```python
from build123d import *

# Parameters (mm, degrees)
SKETCH1_W           = 18
SKETCH1_H           = 14
SKETCH1_R           = 0.5
BOSS_EXTRUDE1_DEPTH = 1
SKETCH2_R           = 4.15
BOSS_EXTRUDE2_DEPTH = 3.75
SKETCH3_W           = 4.05
SKETCH3_H           = 8.25
BOSS_EXTRUDE3_DEPTH = 4.4
SKETCH4_W           = 7.25
SKETCH4_H           = 2
SKETCH4_W_2         = 5.65
SKETCH4_H_2         = 0.9
CUT_EXTRUDE1_DEPTH  = 3
SKETCH5_R           = 3
CUT_EXTRUDE2_DEPTH  = 0.5
CHAMFER1_SIZE       = 0.5


with BuildPart() as part:
    # Sketch1 → Boss-Extrude1 (new body)
    with BuildSketch(Plane(origin=(0, 0, 0), x_dir=(1, 0, 0), z_dir=(0, 1, 0))):
        with Locations((9, 7)):
            Rectangle(SKETCH1_W, SKETCH1_H)
        with Locations(Location((16.5, 12.5, 0), (0, 0, 270))):
            Circle(SKETCH1_R, mode=Mode.SUBTRACT)
        with Locations(Location((16.5, 1.5, 0), (0, 0, 270))):
            Circle(SKETCH1_R, mode=Mode.SUBTRACT)
    extrude(amount=BOSS_EXTRUDE1_DEPTH)

    # Sketch2 → Boss-Extrude2 (add)
    with BuildSketch(Plane(origin=(0, 1, 0), x_dir=(1, 0, 0), z_dir=(0, 1, 0))):
        with Locations(Location((5, 7, 0), (0, 0, 90))):
            Circle(SKETCH2_R)
    extrude(amount=BOSS_EXTRUDE2_DEPTH)

    # Sketch3 → Boss-Extrude3 (add)
    with BuildSketch(Plane(origin=(0, 0, 0), x_dir=(-1, 0, 0), z_dir=(0, -1, 0))):
        with Locations((-15.125, 7)):
            Rectangle(SKETCH3_W, SKETCH3_H)
    extrude(amount=BOSS_EXTRUDE3_DEPTH)

    # Sketch4 → Cut-Extrude1 (cut)
    with BuildSketch(Plane(origin=(17.15, 0, 0), x_dir=(0, 0, -1), z_dir=(1, 0, 0))):
        with Locations((7, -1.5)):
            Rectangle(SKETCH4_W, SKETCH4_H)
        with Locations((7, -3.45)):
            Rectangle(SKETCH4_W_2, SKETCH4_H_2)
    extrude(amount=-CUT_EXTRUDE1_DEPTH, mode=Mode.SUBTRACT)

    # Sketch5 → Cut-Extrude2 (cut)
    with BuildSketch(Plane(origin=(0, 4.75, 0), x_dir=(1, 0, 0), z_dir=(0, 1, 0))):
        with Locations(Location((5, 7, 0), (0, 0, 270))):
            Circle(SKETCH5_R)
    extrude(amount=-CUT_EXTRUDE2_DEPTH, mode=Mode.SUBTRACT)

    # Chamfer1
    chamfer1_edges = [part.edges().sort_by_distance(p)[0] for p in [
        (5, 4.75, -2.85),
    ]]
    chamfer(chamfer1_edges, length=CHAMFER1_SIZE)

    # Sketch7 → Revolve2 (revolve)
    with BuildSketch(Plane.XY.offset(-7)):
        with BuildLine():
            add(Edge.make_bspline(
                [(2.090335023, 4.232825991), (3.350844408, 5.324759463), (4.998474219, 5.209553412)],
                knots=[0, 0, 0, 1, 1, 1], degree=2))
            Line((4.998474219, 5.209553412), (4.998474219, 4.232825991))
            Line((4.998474219, 4.232825991), (2.090335023, 4.232825991))
        make_face()
    revolve(axis=Axis((4.998474219, 4.232825991, -7), (0, 1, 0)))


solid = part.part
```
Can you work these out from the model? Positions are in its coordinate system, mm. A direction names the side the tool comes from. Coordinates: 2 decimals unless noted, no trailing zeros. Order: outer loops, then holes, each group sorted by start corner. A loop starts at its lowest first (then second) coordinate and runs counter-clockwise, first axis right, second up. Notation, with made-up numbers: (33.5, 21) -> (56.5, 21) arc R25 cw to (56.5, 35) -> close; hole circle Ø4 at (-3.5, -37.75). An arc over 180 degrees is marked (long way). Write each question's results on one line, items separated by ' | '.
Item 1: I want a section at B-B, the plane z = -1.5. Write out the boundary of the cut face in (x, y).
Results are:
outline: (0, 0) -> (16, 0) -> (16, 1) -> (0, 1) -> close; (17, 0) -> (18, 0) -> (18, 1) -> (17, 1) -> close
Item 2: I'm going to push flat-ended pins straight in: pin 1 Ø5 at (x, z) = (4.5, -12.5) entering from -Y; pin 2 Ø3 at (x, y) = (15.5, -2) entering from -Z (3 decimals); pin 3 Ø0.7 at (y, z) = (-3.5, -8.5) entering from +X; pin 4 Ø2 at (y, z) = (-3, -1.5) entering from +X. Where does each tip first touch, or does it pass through?
Results are:
pin 1: y = 0 | pin 2: z = -11.125 | pin 3: x = 14.15 | pin 4: through
Item 3: I want a section at C-C, the plane y = -2.25. Write out the boundary of the cut face in (x, z) (3 decimals).
Results are:
outline: (13.1, -11.125) -> (17.15, -11.125) -> (17.15, -10.625) -> (14.15, -10.625) -> (14.15, -3.375) -> (17.15, -3.375) -> (17.15, -2.875) -> (13.1, -2.875) -> close
Item 4: If we mould it in two halves opening along Z, with no side actions, what happens to faces 6 (the face through (16, -3.9, -7)), 7 (the face through (11, 1, -7)), 8 (the face through (14.15, -3.4, -7)), 9 (the face through (15, -2, -11.125))? For each: +Z half, -Z half, draft (parallel to the pull), parting line (faces both ways), or undercut.
Results are:
face 6: undercut | face 7: draft | face 8: undercut | face 9: -Z half
Item 5: I want a section at D-D, the plane x = 10. Write out the boundary of the cut face in (y, z).
Results are:
outline: (0, -14) -> (1, -14) -> (1, 0) -> (0, 0) -> close
Item 6: If I drill on line 1 along X through (y, z) = (0.6, -1.5); line 2 along Y through (x, z) = (16.75, -7.25); line 3 along Z through (x, y) = (15.25, -2.25) (3 decimals), over which ranges is the centre line in solid material (lowest first)?
Results are:
line 1: 0 to 16, 17 to 18 | line 2: -4.4 to -3.9, -3 to -2.5, -0.5 to 1 | line 3: -11.125 to -10.625, -3.375 to -2.875
Item 7: I want a section at A-A, the plane x = 16.5. Write out the boundary of the cut face in (y, z) (3 decimals).
Results are:
outline: (-4.4, -11.125) -> (0, -11.125) -> (0, -12) -> (1, -12) -> (1, -2) -> (0, -2) -> (0, -2.875) -> (-4.4, -2.875) -> close; (0, -14) -> (1, -14) -> (1, -13) -> (0, -13) -> close; (0, -1) -> (1, -1) -> (1, 0) -> (0, 0) -> close; hole (-3.9, -9.825) -> (-3, -9.825) -> (-3, -4.175) -> (-3.9, -4.175) -> close; hole (-2.5, -10.625) -> (-0.5, -10.625) -> (-0.5, -3.375) -> (-2.5, -3.375) -> close
Item 8: Which directions (+Z, -Z, +X, -X, +Y, -Y) give clear straight access to the entire face, cutting with the end or side of a thin tool? Please do faces 1 (the face through (15, -2, -2.875)), 2 (the face through (16.996, 0.493, -12.565)), 3 (the face through (8.9, 0.5, 0)), 4 (the face through (9.05, 2.6, -6.1)), 5 (the face through (16, -0.5, -7)).
Results are:
face 1: +Z, +X, -X, -Y | face 2: +Y, -Y | face 3: +Z, +X, -X, +Y, -Y | face 4: +Y | face 5: +X
